Part model, mm, in its own coordinate system. A direction names the side the tool comes from. Give positions to 0.01 mm unless a question says otherwise; leave off trailing zeros. Write each loop counter-clockwise with the first axis right and the second up, starting at its lowest first coordinate (ties: lowest second). Pieces come first, ordered by that corner, then holes.
Autodesk Inventor part; units mm, degrees
ref_plane "YZ Plane" through (0, 0, 0) normal (1, 0, 0) x (0, 1, 0)
ref_plane "XZ Plane" through (0, 0, 0) normal (0, 1, 0) x (-1, 0, 0)
ref_plane "XY Plane" through (0, 0, 0) normal (0, 0, 1) x (1, 0, 0)
sketch "Sketch1" plane through (0, 0, 0) normal (0, 1, 0) x (-1, 0, 0)
  line L0 (1.5, 0) -> (51, 0)
  line L1 (52.5, 1.5) -> (52.5, 133)
  line L2 (51, 134.5) -> (1.5, 134.5)
  line L3 (0, 133) -> (0, 1.5)
  arc A0 (52.5, 133) -> (51, 134.5) centre (51, 133) ccw
  arc A1 (51, 0) -> (52.5, 1.5) centre (51, 1.5) ccw
  arc A2 (0, 1.5) -> (1.5, 0) centre (1.5, 1.5) ccw
  arc A3 (1.5, 134.5) -> (0, 133) centre (1.5, 133) ccw
  line L4 (57.5, 133) -> (57.5, 1.5)
  arc A4 (51, -5) -> (57.5, 1.5) centre (51, 1.5) ccw
  line L5 (51, -5) -> (1.5, -5)
  arc A5 (-5, 1.5) -> (1.5, -5) centre (1.5, 1.5) ccw
  line L6 (-5, 1.5) -> (-5, 133)
  arc A6 (1.5, 139.5) -> (-5, 133) centre (1.5, 133) ccw
  line L7 (1.5, 139.5) -> (51, 139.5)
  arc A7 (57.5, 133) -> (51, 139.5) centre (51, 133) ccw
  point P0 (0, 0)
  point P1 (52.5, 134.5)
  point P2 (52.5, 0)
  point P3 (0, 134.5)
  dimension "d0" = 52.5
  dimension "d1" = 134.5
  dimension "d2" = 1.5
  dimension "d3" = 5
extrude "Extrusion1" add sketch "Sketch1" against normal blind 4
sketch "Sketch2" plane through (0, -4, 0) normal (0, -1, 0) x (1, 0, 0)
  line L0 (5, 1.5) -> (5, 133)
  arc A0 (5, 133) -> (-1.5, 139.5) centre (-1.5, 133) ccw
  line L1 (-1.5, 139.5) -> (-51, 139.5)
  arc A1 (-51, 139.5) -> (-57.5, 133) centre (-51, 133) ccw
  line L2 (-57.5, 133) -> (-57.5, 1.5)
  arc A2 (-57.5, 1.5) -> (-51, -5) centre (-51, 1.5) ccw
  line L3 (-51, -5) -> (-1.5, -5)
  arc A3 (-1.5, -5) -> (5, 1.5) centre (-1.5, 1.5) ccw
  arc A4 (-1.5, 0) -> (0, 1.5) centre (-1.5, 1.5) ccw
  line L4 (-1.5, 0) -> (-51, 0)
  arc A5 (-52.5, 1.5) -> (-51, 0) centre (-51, 1.5) ccw
  line L5 (-52.5, 1.5) -> (-52.5, 133)
  arc A6 (-51, 134.5) -> (-52.5, 133) centre (-51, 133) ccw
  line L6 (-51, 134.5) -> (-1.5, 134.5)
  arc A7 (0, 133) -> (-1.5, 134.5) centre (-1.5, 133) ccw
  line L7 (0, 133) -> (0, 1.5)
  line L8 (23.75, 117.25) -> (-76.25, 117.25) construction
  line L9 (-76.25, 117.25) -> (-76.25, 17.25) construction
  line L10 (-76.25, 17.25) -> (23.75, 17.25) construction
  line L11 (23.75, 17.25) -> (23.75, 117.25) construction
  circle A8 centre (23.75, 117.25) radius 2.75
  arc A9 (23.75, 107.5) -> (23.75, 127) centre (23.75, 117.25) ccw
  line L12 (5, 1.5) -> (5, 133)
  line L13 (5, 127) -> (23.75, 127)
  line L14 (5, 107.5) -> (23.75, 107.5)
  line L15 (23.75, 67.25) -> (-76.25, 67.25) construction
  line L16 (-26.25, 67.25) -> (-26.25, 117.25) construction
  circle A10 centre (23.75, 17.25) radius 2.75
  arc A11 (23.75, 7.5) -> (23.75, 27) centre (23.75, 17.25) ccw
  line L17 (5, 7.5) -> (23.75, 7.5)
  line L18 (5, 27) -> (23.75, 27)
  circle A12 centre (-76.25, 117.25) radius 2.75
  arc A13 (-76.25, 127) -> (-76.25, 107.5) centre (-76.25, 117.25) ccw
  line L19 (-57.5, 127) -> (-76.25, 127)
  line L20 (-57.5, 107.5) -> (-76.25, 107.5)
  arc A14 (-76.25, 27) -> (-76.25, 7.5) centre (-76.25, 17.25) ccw
  circle A15 centre (-76.25, 17.25) radius 2.75
  line L21 (-57.5, 7.5) -> (-76.25, 7.5)
  line L22 (-57.5, 27) -> (-76.25, 27)
  point P0 (0, 0)
  dimension "d6" = 100
  dimension "d7" = 100
  dimension "d8" = 62.5
  dimension "d9" = 144.5
  dimension "d10" = 18.75
  dimension "d11" = 22.25
  dimension "d12" = 5.5
  dimension "d13" = 7
extrude "Extrusion2" add sketch "Sketch2" along normal blind 4 contours A3 L3 A2 L2 A1 L1 A0 L0 | L0 L18 A11 L17 | L0 L13 A9 L14 | L21 A14 L22 L2 | L20 A13 L19 L2 | L4 A5 L5 A6 L6 A7 L7 A4
sketch "Sketch3" plane through (0, -4, 0) normal (0, 1, 0) x (1, 0, 0)
  line L0 (-49.575, -131.425) -> (-2.925, -131.425) construction
  line L1 (-2.925, -131.425) -> (-2.925, -3.075) construction
  line L2 (-2.925, -3.075) -> (-49.575, -3.075) construction
  line L3 (-49.575, -3.075) -> (-49.575, -131.425) construction
  line L4 (-49.575, -131.425) -> (-49.575, -134.5) construction
  line L5 (-1.5, -134.5) -> (-51, -134.5) construction
  line L6 (-49.575, -131.425) -> (-52.5, -131.425) construction
  line L7 (-52.5, -1.5) -> (-52.5, -133) construction
  line L8 (-2.925, -3.075) -> (0, -3.075) construction
  line L9 (0, -1.5) -> (0, -133) construction
  line L10 (-2.925, -3.075) -> (-2.925, 0) construction
  line L11 (-51, 0) -> (-1.5, 0) construction
  circle A0 centre (-49.575, -131.425) radius 4
  circle A1 centre (-2.925, -131.425) radius 4
  circle A2 centre (-2.925, -3.075) radius 4
  circle A3 centre (-49.575, -3.075) radius 4
  point P0 (0, 0)
  dimension "d16" = 46.65
  dimension "d17" = 128.35
  dimension "d18" = 8
  dimension "d19" = 8
  dimension "d20" = 8
  dimension "d21" = 8
extrude "Extrusion3" add sketch "Sketch3" along normal blind 2.4
sketch "Sketch4" plane through (0, -1.6, 0) normal (0, 1, 0) x (1, 0, 0)
  line L0 (-47.0168, -134.5) -> (-51, -134.5)
  arc A0 (-47.0168, -134.5) -> (-52.5, -128.6966) centre (-49.575, -131.425) ccw
  line L1 (-52.5, -133) -> (-52.5, -128.6966)
  arc A1 (-52.5, -133) -> (-51, -134.5) centre (-51, -133) ccw
  line L2 (0, -128.6966) -> (0, -133)
  arc A2 (0, -128.6966) -> (-5.4832, -134.5) centre (-2.925, -131.425) ccw
  line L3 (-1.5, -134.5) -> (-5.4832, -134.5)
  arc A3 (-1.5, -134.5) -> (0, -133) centre (-1.5, -133) ccw
  line L4 (-52.5, -5.8034) -> (-52.5, -1.5)
  arc A4 (-52.5, -5.8034) -> (-47.0168, 0) centre (-49.575, -3.075) ccw
  line L5 (-51, 0) -> (-47.0168, 0)
  arc A5 (-51, 0) -> (-52.5, -1.5) centre (-51, -1.5) ccw
  line L6 (-5.4832, 0) -> (-1.5, 0)
  arc A6 (-5.4832, 0) -> (0, -5.8034) centre (-2.925, -3.075) ccw
  line L7 (0, -1.5) -> (0, -5.8034)
  arc A7 (0, -1.5) -> (-1.5, 0) centre (-1.5, -1.5) ccw
  circle A8 centre (-49.575, -131.425) radius 1.5
  arc A9 (-52.5, -5.8034) -> (-47.0168, 0) centre (-49.575, -3.075) ccw
  circle A10 centre (-49.575, -3.075) radius 1.5
  circle A11 centre (-2.925, -3.075) radius 1.5
  arc A12 (0, -128.6966) -> (-5.4832, -134.5) centre (-2.925, -131.425) ccw
  circle A13 centre (-2.925, -131.425) radius 1.5
  point P0 (0, 0)
  dimension "d24" = 3
  dimension "d25" = 3
  dimension "d26" = 3
  dimension "d27" = 3
extrude "Extrusion4" cut sketch "Sketch4" against normal through all contours A8 | A10 | A11 | A13
chamfer "Chamfer1" distance 1 angle 45 4 edges at (-51.075, -1.6, 131.425) (-4.425, -1.6, 131.425) (-4.425, -1.6, 3.075) (-51.075, -1.6, 3.075)
equation "\"d10\" = -0.5 * d8 + 0.5 * d6"
equation "\"d11\" = -0.5 * d7 + 0.5 * d9"
equation "\"d19\" = d18"
equation "\"d20\" = d18"
equation "\"d21\" = d18"
equation "\"d25\" = d24"
equation "\"d26\" = d24"
equation "\"d27\" = d24"
properties part number "Elegoo 8 Channel Relay Module"
1) Two-plate mould, pull along Z, no slides. Class faces 1 (the face through (14, -6, 27)), 2 (the face through (3.045, -3.944, 137.646)), 3 (the face through (3.146, -3.944, -3.045)): +Z half, -Z half, draft (parallel to the pull), parting line (faces both ways), or undercut.
Answers follow:
face 1: undercut
face 2: +Z half
face 3: -Z half
2) Saw through at A-A, the plane z = 17.25. Write the cut outline in (x, y), then the cut area to 3 significant figures.
Answers follow:
outline: (-86, -8) - (-79, -8) - (-79, -4) - (-86, -4) - close; (-73.5, -8) - (21, -8) - (21, -4) - (5, -4) - (5, 0) - (0, 0) - (0, -4) - (-52.5, -4) - (-52.5, 0) - (-57.5, 0) - (-57.5, -4) - (-73.5, -4) - close; (26.5, -8) - (33.5, -8) - (33.5, -4) - (26.5, -4) - close
area: 474 mm2
3) 3-axis set-ups, long thin cutter, end or side, ignore diameter. For faces 4 (the face through (14, -6, 127)), 5 (the face through (-67, -6, 107.5)), 6 (the face through (-47.5, -1.6, 5.1)): which of +Z, -Z, +X, -X, +Y, -Y reach the whole face in a straight line?
Answers follow:
face 4: +Z, +X, +Y, -Y
face 5: -X, +Y, -Y
face 6: +Y
4) Pin check, flat tips, straight feed: pin 1 Ø2 at (x, y) = (-71.5, -7) entering from -Z; pin 2 Ø2 at (x, y) = (11, -5.5) entering from +Z; pin 3 Ø4.5 at (x, z) = (23.75, 17.25) entering from -Y; pin 4 Ø1.5 at (x, y) = (3.5, -2.5) entering from -Z. Stop position of each tip, or through.
Answers follow:
pin 1: stops at z = 7.5
pin 2: stops at z = 127
pin 3: passes through
pin 4: stops at z = -3.42
5) Saw through at C-C, the plane z = 92.5. Write the cut outline in (x, y), then the cut area to 3 significant figures.
Answers follow:
outline: (-57.5, -8) - (5, -8) - (5, 0) - (0, 0) - (0, -4) - (-52.5, -4) - (-52.5, 0) - (-57.5, 0) - close
area: 290 mm2
6) Wall check: L1, parallel to Z at x = -76.25, y = -6.8; L2, parallel to Z at x = -2.5, y = -2.75; L3, parallel to X at y = -0.75, z = 56.5. Give the ranges that are in metal, low to high.
Answers follow:
L1: z = 7.5 to 14.5, 20 to 27, 107.5 to 114.5, 120 to 127
L2: z = -5 to 1.64, 4.51 to 7.05, 127.45 to 129.99, 132.86 to 139.5
L3: x = -57.5 to -52.5, 0 to 5
7) Saw through at B-B, the plane x = -65.5. Write the cut outline in (y, z), then the cut area to 3 significant figures.
Answers follow:
outline: (-8, 7.5) - (-4, 7.5) - (-4, 27) - (-8, 27) - close; (-8, 107.5) - (-4, 107.5) - (-4, 127) - (-8, 127) - close
area: 156 mm2
8) Saw through at D-D, the plane y = -6.5. Count the separate pieces of the cut face and the enclosed holes in it, then the cut area to 3 significant figures.
Answers follow:
separate pieces: 1
enclosed holes: 8
area: 10,900 mm2
